```python
from build123d import *

# Parameters (mm, degrees)
SKETCH1_R           = 1.1
BOSS_EXTRUDE1_DEPTH = 5.8
SKETCH2_W           = 0.791647492
SKETCH2_H           = 0.74846672
BOSS_EXTRUDE2_DEPTH = 4


with BuildPart() as part:
    # Sketch1 → Boss-Extrude1 (new body)
    with BuildSketch(Plane.XY):
        with BuildLine():
            Line((0, 6.5), (11.115162843, 9.478298908))
            Line((11.115162843, 9.478298908), (10.79107709, 10.687803405))
            ThreePointArc((10.79107709, 10.687803405), (11.078349161, 15.423518447), (13.684925248, 11.459267786))
            Line((13.684925248, 11.459267786), (14.070629242, 10.011394697))
            Line((14.070629242, 10.011394697), (0.965925826, 6.5))
            Line((0.965925826, 6.5), (12.8, 6.5))
            Line((12.8, 6.5), (12.8, 0))
            Line((12.8, 0), (0, 0))
            Line((0, 0), (0, 6.5))
        make_face()
        with Locations((3.3, 1.5)):
            Circle(SKETCH1_R, mode=Mode.SUBTRACT)
        with Locations((9.5, 1.5)):
            Circle(SKETCH1_R, mode=Mode.SUBTRACT)
    extrude(amount=BOSS_EXTRUDE1_DEPTH)

    # Sketch2 → Boss-Extrude2 (add)
    with BuildSketch(Plane.XZ):
        with Locations((6.397743587, 2.872700046)):
            Rectangle(SKETCH2_W, SKETCH2_H)
        with Locations((1.317743587, 2.872700046)):
            Rectangle(SKETCH2_W, SKETCH2_H)
        with Locations((11.477743587, 2.872700046)):
            Rectangle(SKETCH2_W, SKETCH2_H)
    extrude(amount=BOSS_EXTRUDE2_DEPTH)


solid = part.part
```
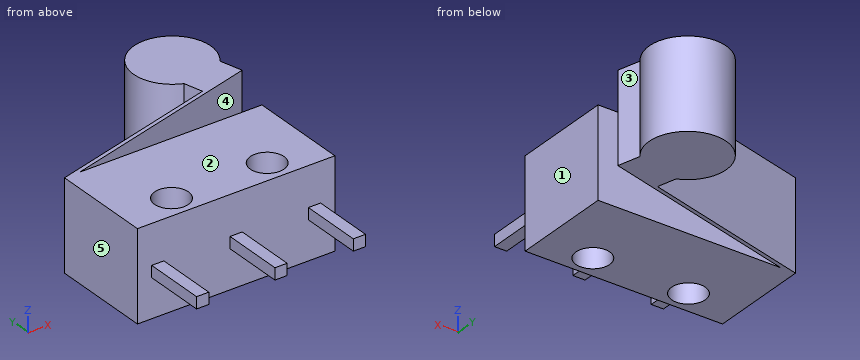
Source: CAD feature listing. Evaluate the final solid. Frame: model axes, mm. Face numbers are marked on the shaded views. A direction names the side the tool comes from. Round coordinates to 2 decimals unless told otherwise and drop trailing zeros. Order: outer loops, then holes, each group sorted by start corner. A loop starts at its lowest first (then second) coordinate and runs counter-clockwise, first axis right, second up. Notation, with made-up numbers: (-30, 31.5) -> (10, 31.5) arc R16 cw to (10, 56.5) -> close; hole circle Ø7 at (28.25, 41). An arc over 180 degrees is marked (long way). One line per item, written item: value. Start each with the question number.
Q1. Section query C-C (x = 9.5). Return the cut outline in (y, z).
Q2. Draft query along Y for the marked faces 4 and 5. Return one class per face: pulls with the +Y half, pulls with the -Y half, needs draft (parallel to the pull), parting line crosses it, or undercut.
Q3. Pin query (flat end, axial travel): pin 1 (0.6 mm diameter, centred on x = 6.5, y = -1, fed in from -Z); pin 2 (3 mm diameter, centred on x = 9.5, y = 1.5, fed in from -Z); pin 3 (3 mm diameter, centred on x = 5.5, z = 4.5, fed in from +Y); pin 4 (0.9 mm diameter, centred on x = 1.5, y = -1.5, fed in from +Z). Return the tip coordinate at first contact, or that it passes through.
Q4. Section query A-A (y = 1.5). Return the cut outline in (x, z), plus the area to 3 significant figures.
Q5. Section query B-B (z = 2.8). Return the cut outline in (x, y).
Q6. Material intervals for probe 1 along Y at (x, z) = (3.3, 2.15); probe 2 along Y at (x, z) = (9.5, 3.05); probe 3 along X at (y, z) = (2, 2.45), sorted ascending.
Q7. Section query D-D (x = 7.25). Return the cut outline in (y, z).
Q8. Access query for the marked faces 1, 2 and 3. Directions: +Z, -Z, +X, -X, +Y, -Y. A direction counts if a zero-diameter tool reaches every point of the face in a straight line with its end or side. Return the directions, or none.
Findings below:
1. outline: (0, 0) -> (0.4, 0) -> (0.4, 5.8) -> (0, 5.8) -> close; (2.6, 0) -> (6.5, 0) -> (6.5, 5.8) -> (2.6, 5.8) -> close; (8.79, 0) -> (9.05, 0) -> (9.05, 5.8) -> (8.79, 5.8) -> close; (11.86, 0) -> (14.15, 0) -> (14.15, 5.8) -> (11.86, 5.8) -> close
2. face 4: undercut
2. face 5: needs draft
3. pin 1: z = 2.5
3. pin 2: z = 0
3. pin 3: y = 8.38
3. pin 4: z = 3.25
4. outline: (0, 0) -> (2.2, 0) -> (2.2, 5.8) -> (0, 5.8) -> close; (4.4, 0) -> (8.4, 0) -> (8.4, 5.8) -> (4.4, 5.8) -> close; (10.6, 0) -> (12.8, 0) -> (12.8, 5.8) -> (10.6, 5.8) -> close
4. area: 48.7 mm²
5. outline: (0, 0) -> (0.92, 0) -> (0.92, -4) -> (1.71, -4) -> (1.71, 0) -> (6, 0) -> (6, -4) -> (6.79, -4) -> (6.79, 0) -> (11.08, 0) -> (11.08, -4) -> (11.87, -4) -> (11.87, 0) -> (12.8, 0) -> (12.8, 6.5) -> (0.97, 6.5) -> (14.07, 10.01) -> (13.68, 11.46) arc R2.5 ccw (long way) to (10.79, 10.69) -> (11.12, 9.48) -> (0, 6.5) -> close; hole circle Ø2.2 at (3.3, 1.5); hole circle Ø2.2 at (9.5, 1.5)
6. probe 1: 0 to 0.4, 2.6 to 6.5, 7.13 to 7.38
6. probe 2: 0 to 0.4, 2.6 to 6.5, 8.79 to 9.05, 11.86 to 14.15
6. probe 3: 0 to 2.32, 4.28 to 8.52, 10.48 to 12.8
7. outline: (0, 0) -> (6.5, 0) -> (6.5, 5.8) -> (0, 5.8) -> close; (8.18, 0) -> (8.44, 0) -> (8.44, 5.8) -> (8.18, 5.8) -> close
8. face 1: +Z, -Z, +X, -Y
8. face 2: +Z, +X, -X, +Y, -Y
8. face 3: +Z, -Z, +X
